```python
from build123d import *

# Parameters (mm, degrees)
BOSS_EXTRUDE1_DEPTH = 17
SKETCH2_R           = 2
CUT_EXTRUDE1_DEPTH  = 89.658793805
CUT_EXTRUDE2_START  = -30
SKETCH3_R           = 75.542453457
SKETCH3_R_2         = 60
CUT_EXTRUDE2_DEPTH  = 30


with BuildPart() as part:
    # Sketch1 → Boss-Extrude1 (new body)
    with BuildSketch(Plane.XY):
        with BuildLine():
            ThreePointArc((59.924052039, 3.017944215), (-60, 0), (59.924052039, -3.017944215))
            ThreePointArc((59.924052039, -3.017944215), (63.018899696, 0), (59.924052039, 3.017944215))
        make_face()
        with BuildLine():
            ThreePointArc((45.423295455, -2.640876758), (47, 0), (45.423295455, 2.640876758))
            ThreePointArc((45.423295455, 2.640876758), (45.266554214, 4.60315865), (45.025082511, 6.556824297))
            ThreePointArc((45.025082511, 6.556824297), (46.037907239, 9.461030444), (43.961873345, 11.730460008))
            ThreePointArc((43.961873345, 11.730460008), (43.413336166, 13.621022095), (42.783537399, 15.486088195))
            ThreePointArc((42.783537399, 15.486088195), (43.191017146, 18.53472519), (40.700646975, 20.339796847))
            ThreePointArc((40.700646975, 20.339796847), (39.782771035, 22.081239295), (38.79042924, 23.781349823))
            ThreePointArc((38.79042924, 23.781349823), (38.575881737, 26.849606109), (35.773131337, 28.116420013))
            ThreePointArc((35.773131337, 28.116420013), (34.523494583, 29.637447964), (33.209236349, 31.103000194))
            ThreePointArc((33.209236349, 31.103000194), (32.381445197, 34.065261), (29.381059498, 34.741953641))
            ThreePointArc((29.381059498, 34.741953641), (27.850822206, 35.980296031), (26.268453421, 37.151290083))
            ThreePointArc((26.268453421, 37.151290083), (24.861308485, 39.886280102), (21.786123631, 39.945147604))
            ThreePointArc((21.786123631, 39.945147604), (20.037933896, 40.85010655), (18.252236923, 41.678601792))
            ThreePointArc((18.252236923, 41.678601792), (16.323346884, 44.074350211), (13.299261303, 43.512982532))
            ThreePointArc((13.299261303, 43.512982532), (11.404690218, 44.047508908), (9.488771701, 44.499586645))
            ThreePointArc((9.488771701, 44.499586645), (7.117105543, 46.458011243), (4.267925654, 45.299390841))
            ThreePointArc((4.267925654, 45.299390841), (2.304537182, 45.441601076), (0.336835051, 45.498753193))
            ThreePointArc((0.336835051, 45.498753193), (-2.380510935, 46.939675837), (-4.938139372, 45.231236768))
            ThreePointArc((-4.938139372, 45.231236768), (-6.889963876, 44.975308757), (-8.828891666, 44.63519544))
            ThreePointArc((-8.828891666, 44.63519544), (-11.780669016, 45.499624587), (-13.942036392, 43.311310546))
            ThreePointArc((-13.942036392, 43.311310546), (-15.802389004, 42.667722013), (-17.633162521, 41.94426754))
            ThreePointArc((-17.633162521, 41.94426754), (-20.698525123, 42.19681336), (-22.375144804, 39.618214182))
            ThreePointArc((-22.375144804, 39.618214182), (-24.06786247, 38.613313716), (-25.715529631, 37.5361364))
            ThreePointArc((-25.715529631, 37.5361364), (-28.76898118, 37.166459636), (-29.892212159, 34.303143475))
            ThreePointArc((-29.892212159, 34.303143475), (-31.347994818, 32.978071819), (-32.745099935, 31.591271425))
            ThreePointArc((-32.745099935, 31.591271425), (-35.661631767, 30.614506688), (-36.185488836, 27.583698043))
            ThreePointArc((-36.185488836, 27.583698043), (-37.344736575, 25.992703787), (-38.434082002, 24.353056085))
            ThreePointArc((-38.434082002, 24.353056085), (-41.094290959, 22.809192239), (-40.997327348, 19.734972772))
            ThreePointArc((-40.997327348, 19.734972772), (-41.812580429, 17.943191408), (-42.549568235, 16.117823769))
            ThreePointArc((-42.549568235, 16.117823769), (-44.844545051, 14.07006678), (-44.130730462, 11.078295397))
            ThreePointArc((-44.130730462, 11.078295397), (-44.568612327, 9.159082664), (-44.923070145, 7.222725853))
            ThreePointArc((-44.923070145, 7.222725853), (-46.758858199, 4.754911133), (-45.457416285, 1.968071307))
            ThreePointArc((-45.457416285, 1.968071307), (-45.5, 0), (-45.457416285, -1.968071307))
            ThreePointArc((-45.457416285, -1.968071307), (-46.758858199, -4.754911133), (-44.923070145, -7.222725853))
            ThreePointArc((-44.923070145, -7.222725853), (-44.568612327, -9.159082664), (-44.130730462, -11.078295397))
            ThreePointArc((-44.130730462, -11.078295397), (-44.844545051, -14.07006678), (-42.549568235, -16.117823769))
            ThreePointArc((-42.549568235, -16.117823769), (-41.812580429, -17.943191408), (-40.997327348, -19.734972772))
            ThreePointArc((-40.997327348, -19.734972772), (-41.094290959, -22.809192239), (-38.434082002, -24.353056085))
            ThreePointArc((-38.434082002, -24.353056085), (-37.344736575, -25.992703787), (-36.185488836, -27.583698043))
            ThreePointArc((-36.185488836, -27.583698043), (-35.661631767, -30.614506688), (-32.745099935, -31.591271425))
            ThreePointArc((-32.745099935, -31.591271425), (-31.347994818, -32.978071819), (-29.892212159, -34.303143475))
            ThreePointArc((-29.892212159, -34.303143475), (-28.76898118, -37.166459636), (-25.715529631, -37.5361364))
            ThreePointArc((-25.715529631, -37.5361364), (-24.06786247, -38.613313716), (-22.375144804, -39.618214182))
            ThreePointArc((-22.375144804, -39.618214182), (-20.698525123, -42.19681336), (-17.633162521, -41.94426754))
            ThreePointArc((-17.633162521, -41.94426754), (-15.802389004, -42.667722013), (-13.942036392, -43.311310546))
            ThreePointArc((-13.942036392, -43.311310546), (-11.780669016, -45.499624587), (-8.828891666, -44.63519544))
            ThreePointArc((-8.828891666, -44.63519544), (-6.889963876, -44.975308757), (-4.938139372, -45.231236768))
            ThreePointArc((-4.938139372, -45.231236768), (-2.380510935, -46.939675837), (0.336835051, -45.498753193))
            ThreePointArc((0.336835051, -45.498753193), (2.304537182, -45.441601076), (4.267925654, -45.299390841))
            ThreePointArc((4.267925654, -45.299390841), (7.117105543, -46.458011243), (9.488771701, -44.499586645))
            ThreePointArc((9.488771701, -44.499586645), (11.404690218, -44.047508908), (13.299261303, -43.512982532))
            ThreePointArc((13.299261303, -43.512982532), (16.323346884, -44.074350211), (18.252236923, -41.678601792))
            ThreePointArc((18.252236923, -41.678601792), (20.037933896, -40.85010655), (21.786123631, -39.945147604))
            ThreePointArc((21.786123631, -39.945147604), (24.861308485, -39.886280102), (26.268453421, -37.151290083))
            ThreePointArc((26.268453421, -37.151290083), (27.850822206, -35.980296031), (29.381059498, -34.741953641))
            ThreePointArc((29.381059498, -34.741953641), (32.381445197, -34.065261), (33.209236349, -31.103000194))
            ThreePointArc((33.209236349, -31.103000194), (34.523494583, -29.637447964), (35.773131337, -28.116420013))
            ThreePointArc((35.773131337, -28.116420013), (38.575881737, -26.849606109), (38.79042924, -23.781349823))
            ThreePointArc((38.79042924, -23.781349823), (39.782771035, -22.081239295), (40.700646975, -20.339796847))
            ThreePointArc((40.700646975, -20.339796847), (43.191017146, -18.53472519), (42.783537399, -15.486088195))
            ThreePointArc((42.783537399, -15.486088195), (43.413336166, -13.621022095), (43.961873345, -11.730460008))
            ThreePointArc((43.961873345, -11.730460008), (46.037907239, -9.461030444), (45.025082511, -6.556824297))
            ThreePointArc((45.025082511, -6.556824297), (45.266554214, -4.60315865), (45.423295455, -2.640876758))
        make_face(mode=Mode.SUBTRACT)
    extrude(amount=BOSS_EXTRUDE1_DEPTH)

    # Sketch2 → Cut-Extrude1 (cut, through all)
    with BuildSketch(Plane.XY.offset(17)):
        with Locations((0, 54)):
            Circle(SKETCH2_R)
        with Locations((38.183766184, 38.183766184)):
            Circle(SKETCH2_R)
        with Locations((54, 0)):
            Circle(SKETCH2_R)
        with Locations((38.183766184, -38.183766184)):
            Circle(SKETCH2_R)
        with Locations((0, -54)):
            Circle(SKETCH2_R)
        with Locations((-38.183766184, -38.183766184)):
            Circle(SKETCH2_R)
        with Locations((-54, 0)):
            Circle(SKETCH2_R)
        with Locations((-38.183766184, 38.183766184)):
            Circle(SKETCH2_R)
    extrude(amount=-CUT_EXTRUDE1_DEPTH, mode=Mode.SUBTRACT)

    # Sketch3 → Cut-Extrude2 (cut)
    with BuildSketch(Plane.XY.offset(17).offset(CUT_EXTRUDE2_START)):
        Circle(SKETCH3_R)
        Circle(SKETCH3_R_2, mode=Mode.SUBTRACT)
    extrude(amount=CUT_EXTRUDE2_DEPTH, mode=Mode.SUBTRACT)


solid = part.part
```
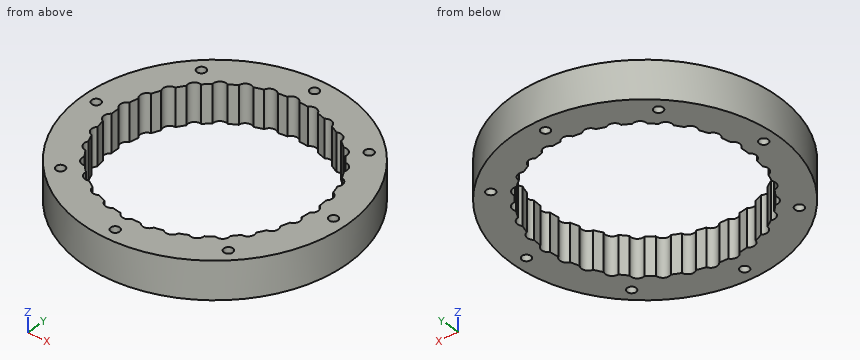
Here's how the part is built. I have some questions about the finished solid (model axes, mm). Give positions to 0.01 mm unless a question says otherwise; leave off trailing zeros. Loops run counter-clockwise (first coordinate to the right, second up) from the corner with the lowest first, then second, coordinate; pieces in that order, holes last. Notation, with made-up numbers: M 80.25,-25 L 105.25,-25 A15 ccw 105.25,-2 Z; hole C 77.5,30.5 d2. An arc over 180 degrees is marked long. Return JSON: item names as keys, results as strings.
Item 1: I'm going to push flat-ended pins straight in: pin 1 Ø3.5 at (x, y) = (-38.18, 38.18) entering from +Z; pin 2 Ø1 at (x, z) = (8.5, 10) entering from +Y; pin 3 Ø1.5 at (x, z) = (-13, 11.5) entering from -Y; pin 4 Ø4 at (y, z) = (-20, 12) entering from +X. Where does each tip first touch, or does it pass through?
A:
{"pin 1": "passes through", "pin 2": "stops at y = 59.46", "pin 3": "stops at y = -58.74", "pin 4": "stops at x = 57.24"}
Item 2: Imagine slicing it at A-A on y = 0. List the corners of the cut face in (x, z) for me, then the cut area to 4 significant figures.
A:
{"outline": "M -60,0 L -56,0 L -56,17 L -60,17 Z; M -52,0 L -45.5,0 L -45.5,17 L -52,17 Z; M 47,0 L 52,0 L 52,17 L 47,17 Z; M 56,0 L 60,0 L 60,17 L 56,17 Z", "area": "331.5 mm^2"}
Item 3: Imagine slicing it at B-B on x = 54. List the corners of the cut face in (y, z) for me, then the cut area to 3 significant figures.
A:
{"outline": "M -26.15,0 L -2,0 L -2,17 L -26.15,17 Z; M 2,0 L 26.15,0 L 26.15,17 L 2,17 Z", "area": "821 mm^2"}
Item 4: Imagine slicing it at D-D on z = 9. State how many separate pieces and enclosed holes the cut face has, then the cut area to 3 significant figures.
A:
{"separate pieces": "1", "enclosed holes": "9", "area": "4,530 mm^2"}
Item 5: Please list where these lines run through material, in increasing order: line 1 (Y direction, x = -38, z = 10.5); line 2 (X direction, y = 8.5, z = 6.75); line 3 (Y direction, x = -3.5, z = 12).
A:
{"line 1": "y = -46.43 to -40.18, -36.19 to -25.02, 25.02 to 36.19, 40.18 to 46.43", "line 2": "x = -59.39 to -44.7, 46.08 to 59.39", "line 3": "y = -59.9 to -46.66, 46.66 to 59.9"}
